Geometry check sheet. Reference: the model listing, model coordinates, mm. Face numbers are marked on the shaded views. A direction names the side the tool comes from. Coordinates: 2 decimals unless noted, no trailing zeros. Order: outer loops, then holes, each group sorted by start corner. A loop starts at its lowest first (then second) coordinate and runs counter-clockwise, first axis right, second up. Notation, with made-up numbers: (-2.5, 71) -> (6.5, 71) arc R36 cw to (6.5, 109) -> close; hole circle Ø5 at (61, -11). An arc over 180 degrees is marked (long way). Answer as CSV lines item,"result". Start each with the question number.
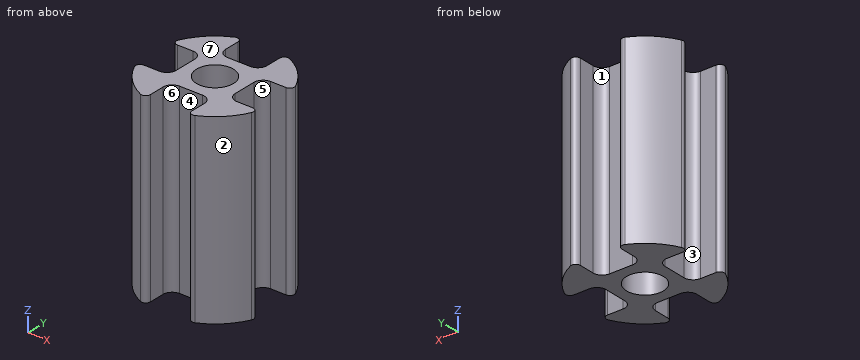
from build123d import *

# Parameters (mm, degrees)
SKETCH_2_R          = 7
EXTRUDE_1_DEPTH     = 20
SKETCH_4_W          = 4.5
SKETCH_4_H          = 3.8
SKETCH_4_W_2        = 3.8
SKETCH_4_H_2        = 4.5
CUT_EXTRUDE_1_DEPTH = 20
SKETCH_5_R          = 2
CUT_EXTRUDE_2_DEPTH = 20
FILLET_1_R          = 1
FILLET_2_R          = 0.5


with BuildPart() as part:
    # 草图2 → 凸台-拉伸1 (new body)
    with BuildSketch(Plane.XY):
        Circle(SKETCH_2_R)
    extrude(amount=EXTRUDE_1_DEPTH)

    # 草图4 → 切除-拉伸1 (cut)
    with BuildSketch(Plane.XY.offset(20)):
        with Locations((0, 5.1)):
            Rectangle(SKETCH_4_W, SKETCH_4_H)
        with Locations((5.1, 0)):
            Rectangle(SKETCH_4_W_2, SKETCH_4_H_2)
        with Locations((0, -5.1)):
            Rectangle(SKETCH_4_W, SKETCH_4_H)
        with Locations((-5.1, 0)):
            Rectangle(SKETCH_4_W_2, SKETCH_4_H_2)
    extrude(amount=-CUT_EXTRUDE_1_DEPTH, mode=Mode.SUBTRACT)

    # 草图5 → 切除-拉伸2 (cut)
    with BuildSketch(Plane.XY.offset(20)):
        Circle(SKETCH_5_R)
    extrude(amount=-CUT_EXTRUDE_2_DEPTH, mode=Mode.SUBTRACT)

    # 圆角1
    fillet_1_edges = [part.edges().sort_by_distance(p)[0] for p in [
        (-2.25, 3.2, 10),
        (2.25, 3.2, 10),
        (3.2, 2.25, 10),
        (3.2, -2.25, 10),
        (2.25, -3.2, 10),
        (-2.25, -3.2, 10),
        (-3.2, -2.25, 10),
        (-3.2, 2.25, 10),
    ]]
    fillet(fillet_1_edges, radius=FILLET_1_R)

    # 圆角2
    fillet_2_edges = [part.edges().sort_by_distance(p)[0] for p in [
        (-2.25, 6.628536792, 10),
        (2.25, 6.628536792, 10),
        (6.628536792, -2.25, 10),
        (6.628536792, 2.25, 10),
        (2.25, -6.628536792, 10),
        (-2.25, -6.628536792, 10),
        (-6.628536792, 2.25, 10),
        (-6.628536792, -2.25, 10),
    ]]
    fillet(fillet_2_edges, radius=FILLET_2_R)


solid = part.part
Q1. Sectioned sample at A-A, the plane y = 0. Record the cut outline in (x, z), then the cut area to 3 significant figures.
Q2. Thickness scan on L1, parallel to Y at x = 0, z = 11.75; L2, parallel to X at y = -4.5, z = 3; L3, parallel to Y at x = 5.5, z = 3. Record the ranges inside material, lowest first.
Q3. Access from +Z, -Z, +X, -X, +Y, -Y to the whole of each face (thin tool, end or side, straight path). Record for the marked faces 1, 2, 3 and 4.
Q4. Release check for a two-part mould opening along Y. For the marked faces 5, 6 and 7 record: released by +Y, released by -Y, zero draft, split by the parting line, or undercut.
Q5. Go/stop test with flat-tipped pins: pin 1 Ø2 at (x, z) = (0, 10.5) entering from +Y; pin 2 Ø1 at (y, z) = (-2, 5.5) entering from -X; pin 3 Ø0.8 at (y, z) = (5, 9.5) entering from -X. Record where each tip stops, or that it passes through.
Geometry results:
1,outline,"(-3.2, 0) -> (-2, 0) -> (-2, 20) -> (-3.2, 20) -> close; (2, 0) -> (3.2, 0) -> (3.2, 20) -> (2, 20) -> close"
1,area,"48.0 mm^2"
2,L1,"y = -3.2 to -2, 2 to 3.2"
2,L2,"x = -5.36 to -2.25, 2.25 to 5.36"
2,L3,"y = -4.33 to -2.25, 2.25 to 4.33"
3,face 1,"+Z, -Z, +Y"
3,face 2,"+Z, -Z, +X, -Y"
3,face 3,"+Z, -Z, -X"
3,face 4,"+Z, -Z, -Y"
4,face 5,"undercut"
4,face 6,"released by -Y"
4,face 7,"zero draft"
5,pin 1,"stops at y = 3.2"
5,pin 2,"stops at x = -6.32"
5,pin 3,"stops at x = -5.28"
